CAD build for the part. Positions are in the model's coordinates, mm. Give positions to 0.01 mm unless a question says otherwise; leave off trailing zeros. Loops run counter-clockwise (first coordinate to the right, second up) from the corner with the lowest first, then second, coordinate; pieces in that order, holes last. Notation, with made-up numbers: (33, -35.75) -> (78, -35.75) arc R12 cw to (78, -16.75) -> close; hole circle Ø8 at (69.25, 49.25). An arc over 180 degrees is marked (long way). Use one line per item in the form item = value.
```python
from build123d import *

# Parameters (mm, degrees)
SKETCH_1_W          = 126
SKETCH_1_H          = 53
EXTRUDE_1_DEPTH     = 3
SKETCH_2_R          = 1.55
SKETCH_2_R_2        = 1.5
CUT_EXTRUDE_1_DEPTH = 10
SKETCH_3_R          = 1.55
CUT_EXTRUDE_2_DEPTH = 10
SKETCH_5_R          = 1.55
CUT_EXTRUDE_5_DEPTH = 10
CUT_EXTRUDE_7_DEPTH = 69.412352686


with BuildPart() as part:
    # 草图1 → 凸台-拉伸1 (new body)
    with BuildSketch(Plane.XY):
        Rectangle(SKETCH_1_W, SKETCH_1_H)
    extrude(amount=EXTRUDE_1_DEPTH)

    # 草图2 → 切除-拉伸1 (cut)
    with BuildSketch(Plane(origin=(0, 0, 0), x_dir=(-1, 0, 0), z_dir=(0, 0, -1))):
        with Locations((56, 21.5)):
            Circle(SKETCH_2_R)
        with Locations((-56, 21.5)):
            Circle(SKETCH_2_R_2)
    extrude(amount=-CUT_EXTRUDE_1_DEPTH, mode=Mode.SUBTRACT)

    # 草图3 → 切除-拉伸2 (cut)
    with BuildSketch(Plane.XY.offset(3)):
        with Locations((-56, -8.5)):
            Circle(SKETCH_3_R)
        with Locations((56, -8.5)):
            Circle(SKETCH_3_R)
    extrude(amount=-CUT_EXTRUDE_2_DEPTH, mode=Mode.SUBTRACT)

    # 草图5 → 切除-拉伸5 (cut)
    with BuildSketch(Plane.XY.offset(3)):
        with Locations((56, 3.5)):
            Circle(SKETCH_5_R)
    extrude(amount=-CUT_EXTRUDE_5_DEPTH, mode=Mode.SUBTRACT)

    # 草图6 → 切除-拉伸7 (cut, through all)
    with BuildSketch(Plane.XY.offset(3)):
        Polygon((62.980435582, -3.5), (60, -3.5), (-60, -23.5), (-63, -23.5), (-63, -26.5), (63, -26.5), (63, -3.5), align=None)
    extrude(amount=-CUT_EXTRUDE_7_DEPTH, mode=Mode.SUBTRACT)


solid = part.part
```
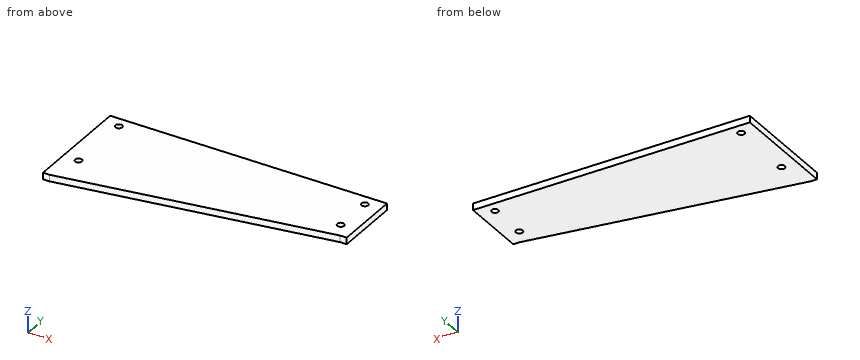
1. Drill centre lines: line 1 (Y direction, x = -56, z = 1.9); line 2 (X direction, y = 20.5, z = 2.2); line 3 (Y direction, x = 56, z = 0.75). Where is each one in solid material? Low to high.
Result sheet:
line_1 = -22.83 to -10.05, -6.95 to 19.95, 23.05 to 26.5
line_2 = -63 to -57.18, -54.82 to 54.88, 57.12 to 63
line_3 = -4.17 to 1.95, 5.05 to 20, 23 to 26.5
2. Cut at B-B, the plane z = 1.4. Write the cut outline in (x, y), then the cut area to 3 significant figures.
Result sheet:
outline = (-63, -23.5) -> (-60, -23.5) -> (60, -3.5) -> (63, -3.5) -> (63, 26.5) -> (-63, 26.5) -> close; hole circle Ø3.1 at (-56, -8.5); hole circle Ø3.1 at (-56, 21.5); hole circle Ø3.1 at (56, 3.5); hole circle Ø3 at (56, 21.5)
area = 5,010 mm^2
3. Drop flat-ended pins along their axis: P1, Ø1.8, axis at x = 56, y = 21.5, coming from the +Z side; P2, Ø3.5, axis at x = -56, y = 21.5, coming from the +Z side; P3, Ø1.5, axis at x = 62, z = 2, coming from the -Y side. Give the stop position or say it passes through.
Result sheet:
P1 = through
P2 = 3
P3 = -3.5
4. Cut at C-C, the plane x = -56. Write the cut outline in (y, z), then the cut area to 3 significant figures.
Result sheet:
outline = (-22.83, 0) -> (-10.05, 0) -> (-10.05, 3) -> (-22.83, 3) -> close; (-6.95, 0) -> (19.95, 0) -> (19.95, 3) -> (-6.95, 3) -> close; (23.05, 0) -> (26.5, 0) -> (26.5, 3) -> (23.05, 3) -> close
area = 129 mm^2
5. Cut at A-A, the plane y = -8.5. Write the cut outline in (x, z).
Result sheet:
outline = (-63, 0) -> (-57.55, 0) -> (-57.55, 3) -> (-63, 3) -> close; (-54.45, 0) -> (30, 0) -> (30, 3) -> (-54.45, 3) -> close
6. Cut at D-D, the plane y = 3.5. Write the cut outline in (x, z), then the cut area to 3 significant figures.
Result sheet:
outline = (-63, 0) -> (54.45, 0) -> (54.45, 3) -> (-63, 3) -> close; (57.55, 0) -> (63, 0) -> (63, 3) -> (57.55, 3) -> close
area = 369 mm^2
